from build123d import *
from build123d.topology import SkipClean

# Parameters (mm, degrees)
CUT_EXTRUDE1_DEPTH      = 5
SKETCH3_R               = 2.5
CUT_EXTRUDE2_DEPTH      = 10
CUT_EXTRUDE4_DEPTH      = 28.349589
CUT_EXTRUDE4_DEPTH_BACK = 28.349589
CUT_EXTRUDE5_REACH      = 29.586
SKETCH5_R               = 4.5


with BuildPart() as part:
    # Sketch1 → Revolve1 (revolve)
    with BuildSketch(Plane.XY, mode=Mode.PRIVATE) as revolve1_sk:
        with BuildLine():
            Line((6, 0), (-26, 0))
            ThreePointArc((-26, 0), (-22.021548, 4.894532), (-16.417424, 2))
            Line((-16.417424, 2), (-5.656854, 2))
            ThreePointArc((-5.656854, 2), (1.014612, 5.913591), (6, 0))
        make_face()
    revolve(revolve1_sk.sketch.rotate(Axis((6.214657, 0, 0), (-1, 0, 0)), 90), axis=Axis((6.214657, 0, 0), (-1, 0, 0)))

    # Sketch2 → Cut-Extrude1 (cut, symmetric)
    with SkipClean():  # the faces are left unmerged after this step: merging them gives an invalid solid
        with BuildSketch(Plane.XY):
            with BuildLine():
                Line((-16.669873, 2.5), (-25.330127, 2.5))
                ThreePointArc((-25.330127, 2.5), (-21, 5), (-16.669873, 2.5))
            make_face()
            with BuildLine():
                Line((-16.669873, -2.5), (-25.330127, -2.5))
                ThreePointArc((-25.330127, -2.5), (-21, -5), (-16.669873, -2.5))
            make_face()
        extrude(amount=CUT_EXTRUDE1_DEPTH, both=True, mode=Mode.SUBTRACT)

    # Sketch3 → Cut-Extrude2 (cut)
    with SkipClean():  # the faces are left unmerged after this step: merging them gives an invalid solid
        with BuildSketch(Plane(origin=(0, 2.5, 0), x_dir=(1, 0, 0), z_dir=(0, 1, 0))):
            with Locations(Location((-21, 0, 0), (0, 0, 270))):
                Circle(SKETCH3_R)
        extrude(amount=-CUT_EXTRUDE2_DEPTH, mode=Mode.SUBTRACT)

    # Sketch4 → Cut-Extrude4 (cut, two sides: drawn at the far end of the back side and taken through both)
    with SkipClean():  # the faces are left unmerged after this step: merging them gives an invalid solid
        with BuildSketch(Plane(origin=(0, 0, 0), x_dir=(1, 0, 0), z_dir=(0, 1, 0)).offset(-CUT_EXTRUDE4_DEPTH_BACK)):
            with BuildLine():
                Line((-5.656854, 2), (5.656854, 2))
                ThreePointArc((5.656854, 2), (0, 6), (-5.656854, 2))
            make_face()
            with BuildLine():
                Line((-5.656854, -2), (5.656854, -2))
                ThreePointArc((5.656854, -2), (0, -6), (-5.656854, -2))
            make_face()
        extrude(amount=CUT_EXTRUDE4_DEPTH + CUT_EXTRUDE4_DEPTH_BACK, mode=Mode.SUBTRACT)

    # Sketch5 → Cut-Extrude5 (cut, up to next)
    with BuildSketch(Plane(origin=(0, 0, -2), x_dir=(-1, 0, 0), z_dir=(0, 0, -1)), mode=Mode.PRIVATE) as cut_extrude5_sk1:
        Circle(SKETCH5_R)
    cut_extrude5_tool1 = extrude(cut_extrude5_sk1.sketch, amount=-CUT_EXTRUDE5_REACH, mode=Mode.PRIVATE) & part.part
    add(cut_extrude5_tool1.solids().sort_by_distance((0, 0, -2))[0], mode=Mode.SUBTRACT)

    # Sketch6 → Cut-Revolve1 (revolve, cut)
    with SkipClean():  # the faces are left unmerged after this step: merging them gives an invalid solid
        with BuildSketch(Plane.XY):
            with BuildLine():
                Line((0, 5), (0, -5))
                ThreePointArc((0, -5), (-5, 0), (0, 5))
            make_face()
        revolve(axis=Axis((0, 8.612845, 0), (0, -1, 0)), mode=Mode.SUBTRACT)


solid = part.part
Work out the finished part from the listing and answer in its coordinate system (mm). A direction names the side the tool comes from. Coordinates: 2 decimals unless noted, no trailing zeros. Order: outer loops, then holes, each group sorted by start corner. A loop starts at its lowest first (then second) coordinate and runs counter-clockwise, first axis right, second up. Notation, with made-up numbers: (-17, 55.5) - (19, 55.5) arc R14 ccw to (19, 71.5) - close; hole circle Ø6 at (39, -20.75). An arc over 180 degrees is marked (long way). Put each result on its own line as item: value. Start each with the question number.
1) Find section C-C (x = -10.5). Give the vertices of the cut face in (y, z).
2) For faces 1 (the flat face through (-23, -2.5, -2)), 2 (the cylindrical face through (-11, 2, 0)), determine the directions among +Z, -Z, +X, -X, +Y, -Y from which every point of the face is accessible in a straight line to the end or side of a thin tool.
3) For a pull along Z with two mould halves and no side action, classify faces 3 (the flat face through (5, 0, 2)), 4 (the flat face through (5, 0, -2)), 5 (the cylindrical face through (-18.52, 0.04, -0.33)), 6 (the flat face through (-23, 2.5, 2)) as released by +Z, released by -Z, zero draft, split by the parting line, or undercut.
4) Find the intervals of material crossed by line 1 (X direction, y = -0.1, z = 0); line 2 (X direction, y = 1.25, z = 0.5); line 3 (Y direction, x = -24, z = 0.5), in increasing order. Write a range as from..to.
5) Find section A-A (z = -1.25). State how many separate pieces and enclosed holes the cut face has, plus the area to 3 significant figures.
6) Flat-ended cylindrical pins translate along their axes: pin 1 (1.5 mm diameter, centred on y = 4.5, z = 1.5, fed in from -X); pin 2 (1.5 mm diameter, centred on y = 1.5, z = 0, fed in from +X); pin 3 (2.5 mm diameter, centred on x = -22, z = 2, fed in from +Y). Find the tip coordinate at first contact, or state that the pin passes through.
Results list:
1. outline: circle Ø4 at (0, 0)
2. face 1: +Z, -Z, -X, -Y
2. face 2: none
3. face 3: released by +Z
3. face 4: released by -Z
3. face 5: undercut
3. face 6: zero draft
4. line 1: x = -26..-23.5, -18.5..-5, 5..6
4. line 2: x = -25.82..-23.45, -18.55..-4.82, 4.82..5.85
4. line 3: y = -2.5..2.5
5. separate pieces: 2
5. enclosed holes: 1
5. area: 91.7 mm^2
6. pin 1: stops at x = -4.48
6. pin 2: stops at x = 5.95
6. pin 3: stops at y = 2.5
